Geometry check sheet. Reference: drawing and pictorial views, mm from the part's lowest x, y, z. Give positions to 0.01 mm unless a question says otherwise; leave off trailing zeros. Write each loop counter-clockwise with the first axis right and the second up, starting at its lowest first coordinate (ties: lowest second). Pieces come first, ordered by that corner, then holes. Notation, with made-up numbers: (26, 54) -> (59, 54) arc R9 ccw to (59, 61) -> close; hole circle Ø9 at (82.25, 34.25). An arc over 180 degrees is marked (long way). Use a Markdown table: item, result. Add a question column.
1. Cross-section at C-C (y = 7.75). Enter the section's corners in (x, z).
2. Cross-section at A-A (z = 10.25). Enter the section's corners in (x, y).
3. Scan lines: probe 1 along Y at (x, z) = (9, 17.5); probe 2 along Z at (x, y) = (19.25, 5.5); probe 3 along Z at (x, y) = (11, 2.5). Record each from-to range of solid material in increasing order. Write a range as [from, to].
4. Cross-section at D-D (z = 21). Enter the section's corners in (x, y), then the cut area to 3 significant figures.
5. Cross-section at B-B (x = 8). Enter the section's corners in (y, z).
6. Gauge pin test, flat ends, axial feed: P1, Ø1.5, axis at x = 13, y = 2.5, coming from the +Z side; P2, Ø1.3, axis at x = 11, y = 2, coming from the +Z side; P3, Ø4, axis at x = 10, y = 6, coming from the +Z side. Record the tip position at first contact, or that the pin passes through.
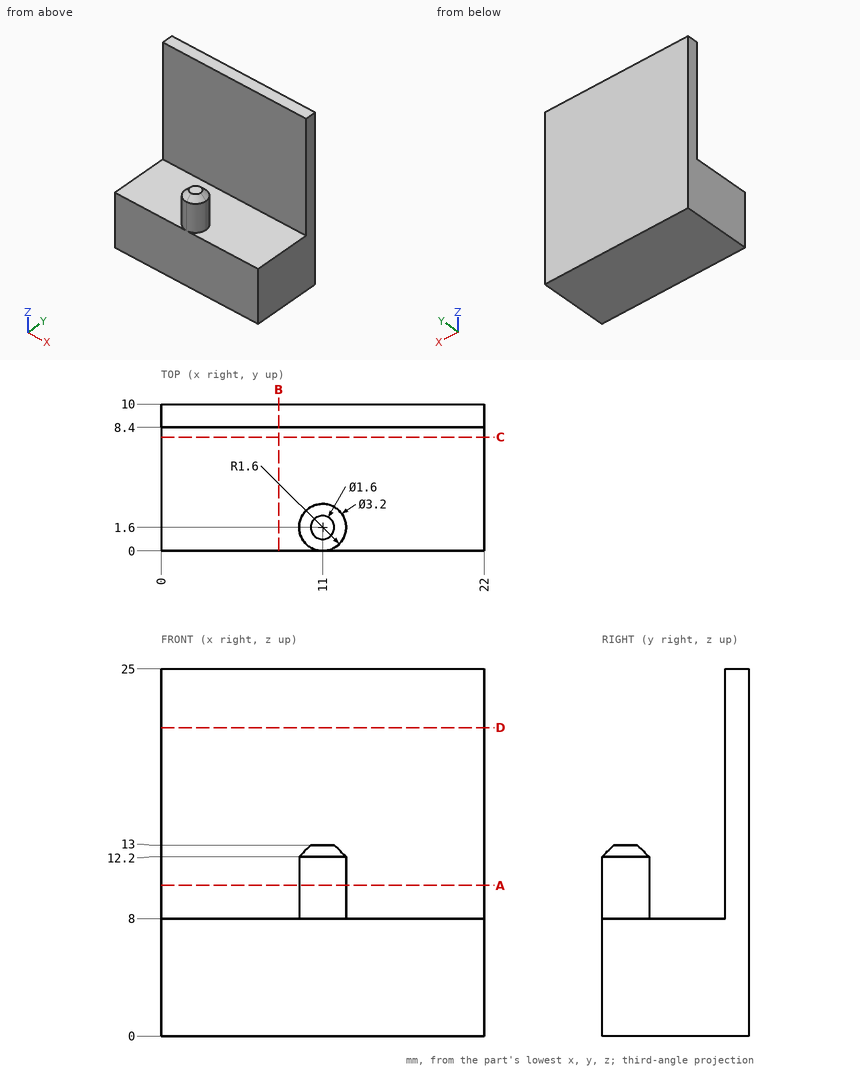
Worked answers:
| question | item | result |
|---|---|---|
| 1 | outline | (0, 0) -> (22, 0) -> (22, 8) -> (0, 8) -> close |
| 2 | outline | (0, 8.4) -> (22, 8.4) -> (22, 10) -> (0, 10) -> close; circle Ø3.2 at (11, 1.6) |
| 3 | probe 1 | y = [8.4, 10] |
| 3 | probe 2 | z = [0, 8] |
| 3 | probe 3 | z = [0, 12.9] |
| 4 | outline | (0, 8.4) -> (22, 8.4) -> (22, 10) -> (0, 10) -> close |
| 4 | area | 35.2 mm² |
| 5 | outline | (0, 0) -> (10, 0) -> (10, 25) -> (8.4, 25) -> (8.4, 8) -> (0, 8) -> close |
| 6 | P1 | stops at z = 12.36 |
| 6 | P2 | stops at z = 13 |
| 6 | P3 | stops at z = 8 |
